Job drawing, mm, ordinate dimensions from the low corner. One solid piece. A direction names the side the tool comes from. Give positions to 0.01 mm unless a question says otherwise; leave off trailing zeros. Order: outer loops, then holes, each group sorted by start corner. A loop starts at its lowest first (then second) coordinate and runs counter-clockwise, first axis right, second up.
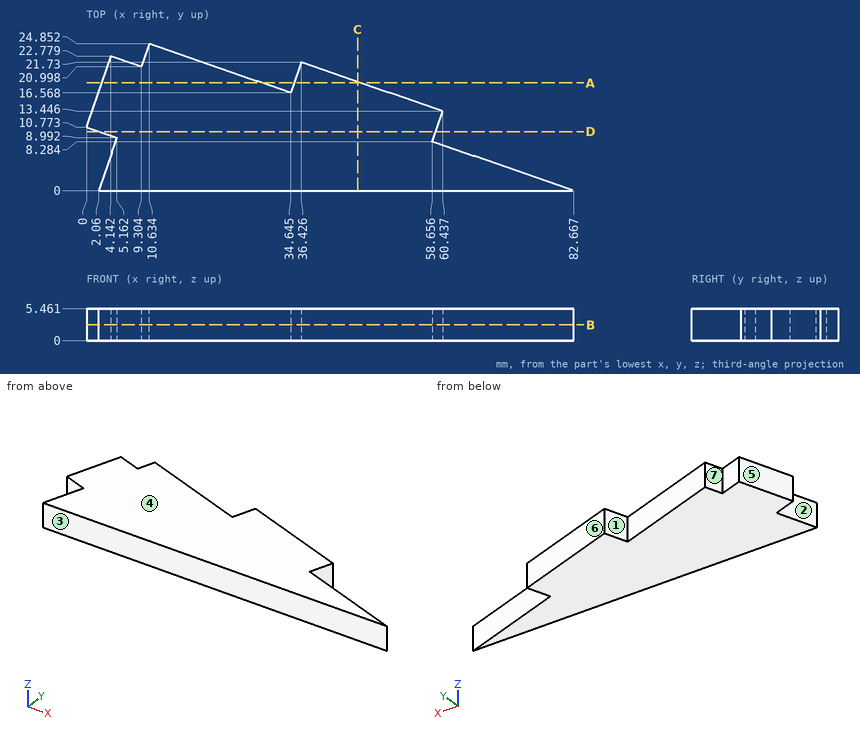
Item 1: Band-saw the part on D-D on y = 10. List the corners of the cut face in (x, z).
Item 2: Drill centre lines: probe 1 along Y at (x, z) = (41, 4.5); probe 2 along Y at (x, z) = (72, 4.2); probe 3 along X at (y, z) = (12.5, 0.8) (1 decimal). Where is each one in solid material? Low to high.
Item 3: Band-saw the part on A-A on y = 18.25. List the corners of the cut face in (x, z) (1 decimal).
Item 4: Drop flat-ended pins along their axis: P1, Ø2, axis at x = 18.5, z = 4, coming from the -Y side; P2, Ø1.5, axis at x = 58, z = 0.5, coming from the +Y side (1 decimal). Give the stop position or say it passes through.
Item 5: Band-saw the part on B-B on z = 2.7. List the corners of the cut face in (x, y) (1 decimal).
Item 6: Which spindle directions (+Z, -Z, +X, -X, +Y, -Y) get a long thin tool onto all of the face, cutting with end or side? Do the marked faces 1, 2 and 3. Say none if no direction does.
Item 7: Band-saw the part on C-C on x = 46. List the corners of the cut face in (y, z), plus the area to 3 significant figures.
Item 8: Pull direction X, two halves, no side cores. Call the marked faces 4, 5, 6 and 7: released by +X, released by -X, zero draft, split by the parting line, or undercut.
Working result:
1. outline: (2.24, 0) - (59.25, 0) - (59.25, 5.46) - (2.24, 5.46) - close
2. probe 1: y = 0 to 20.15
2. probe 2: y = 0 to 3.68
2. probe 3: x = 0.6 to 60.1
3. outline: (2.6, 0) - (29.8, 0) - (29.8, 5.5) - (2.6, 5.5) - close; (35.2, 0) - (46.5, 0) - (46.5, 5.5) - (35.2, 5.5) - close
4. P1: stops at y = 0
4. P2: stops at y = 14.5
5. outline: (0, 10.8) - (5.2, 9) - (2.1, 0) - (82.7, 0) - (58.7, 8.3) - (60.4, 13.4) - (36.4, 21.7) - (34.6, 16.6) - (10.6, 24.9) - (9.3, 21) - (4.1, 22.8) - close
6. face 1: +Z, -Z, +Y
6. face 2: +Z, -Z, -X
6. face 3: +Z, -Z, +X, -X, -Y
7. outline: (0, 0) - (18.43, 0) - (18.43, 5.46) - (0, 5.46) - close
7. area: 101 mm2
8. face 4: zero draft
8. face 5: released by -X
8. face 6: released by +X
8. face 7: undercut
